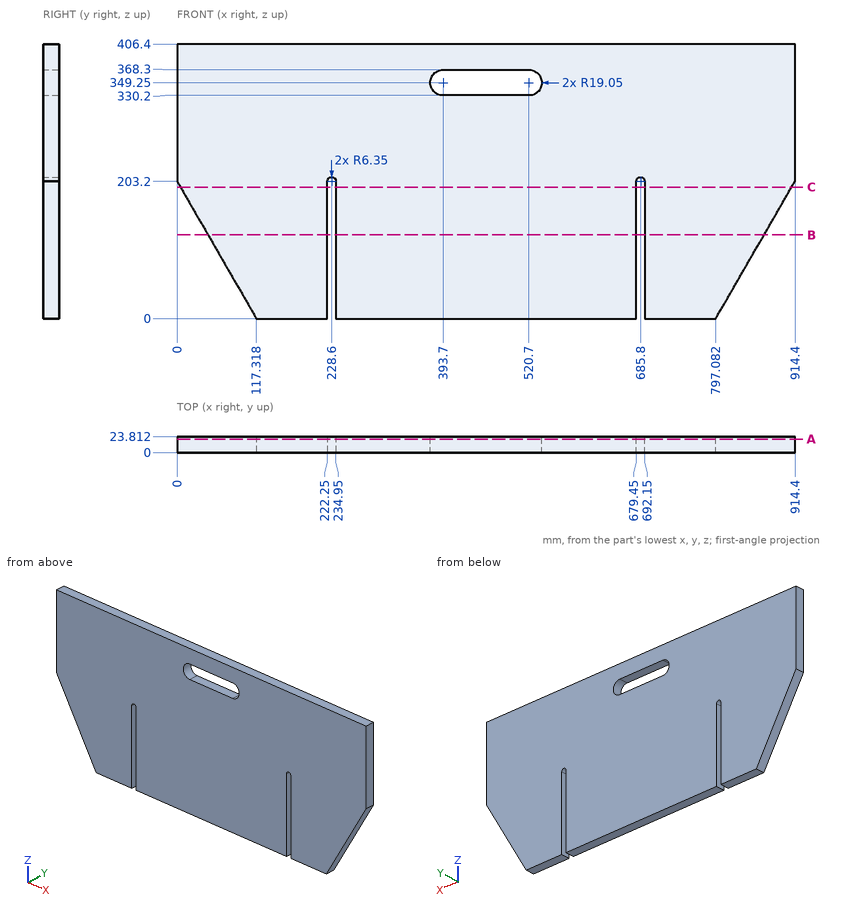
Check sheet for the drawn part. Datum: minimum x, y, z corner. Units: mm. Round coordinates to 2 decimals unless told otherwise and drop trailing zeros. Loops run counter-clockwise (first coordinate to the right, second up) from the corner with the lowest first, then second, coordinate; pieces in that order, holes last.
Item 1: Gauge pin test, flat end, axial feed: pin 1 (12 mm diameter, centred on y = 17, z = 92, fed in from -X). Record the tip position at first contact, or that the pin passes through.
Item 2: Thickness scan on line 1 (X direction, y = 6.5, z = 83); line 2 (Z direction, x = 452, y = 5); line 3 (X direction, y = 12.25, z = 208) (1 decimal). Record the ranges inside material, lowest first.
Item 3: Cross-section at B-B on z = 124. Record the boundary of the cut face in (x, y).
Item 4: Cross-section at C-C on z = 194.5. Record the boundary of the cut face in (x, y), then the cut area to 3 significant figures.
Item 5: Cross-section at A-A on y = 20. Record the boundary of the cut face in (x, z), then the cut area to 3 significant figures.
Answer sheet:
1. pin 1: stops at x = 60.74
2. line 1: x = 69.4 to 222.25, 234.95 to 679.45, 692.15 to 845
2. line 2: z = 0 to 330.2, 368.3 to 406.4
2. line 3: x = 0 to 224.4, 232.8 to 681.6, 690 to 914.4
3. outline: (45.73, 0) - (222.25, 0) - (222.25, 23.81) - (45.73, 23.81) - close; (234.95, 0) - (679.45, 0) - (679.45, 23.81) - (234.95, 23.81) - close; (692.15, 0) - (868.67, 0) - (868.67, 23.81) - (692.15, 23.81) - close
4. outline: (5.02, 0) - (222.25, 0) - (222.25, 23.81) - (5.02, 23.81) - close; (234.95, 0) - (679.45, 0) - (679.45, 23.81) - (234.95, 23.81) - close; (692.15, 0) - (909.38, 0) - (909.38, 23.81) - (692.15, 23.81) - close
4. area: 20,900 mm2
5. outline: (0, 203.2) - (117.32, 0) - (222.25, 0) - (222.25, 203.2) arc R6.35 cw to (234.95, 203.2) - (234.95, 0) - (679.45, 0) - (679.45, 203.2) arc R6.35 cw to (692.15, 203.2) - (692.15, 0) - (797.08, 0) - (914.4, 203.2) - (914.4, 406.4) - (0, 406.4) - close; hole (393.7, 330.2) - (520.7, 330.2) arc R19.05 ccw to (520.7, 368.3) - (393.7, 368.3) arc R19.05 ccw to start
5. area: 337,000 mm2
